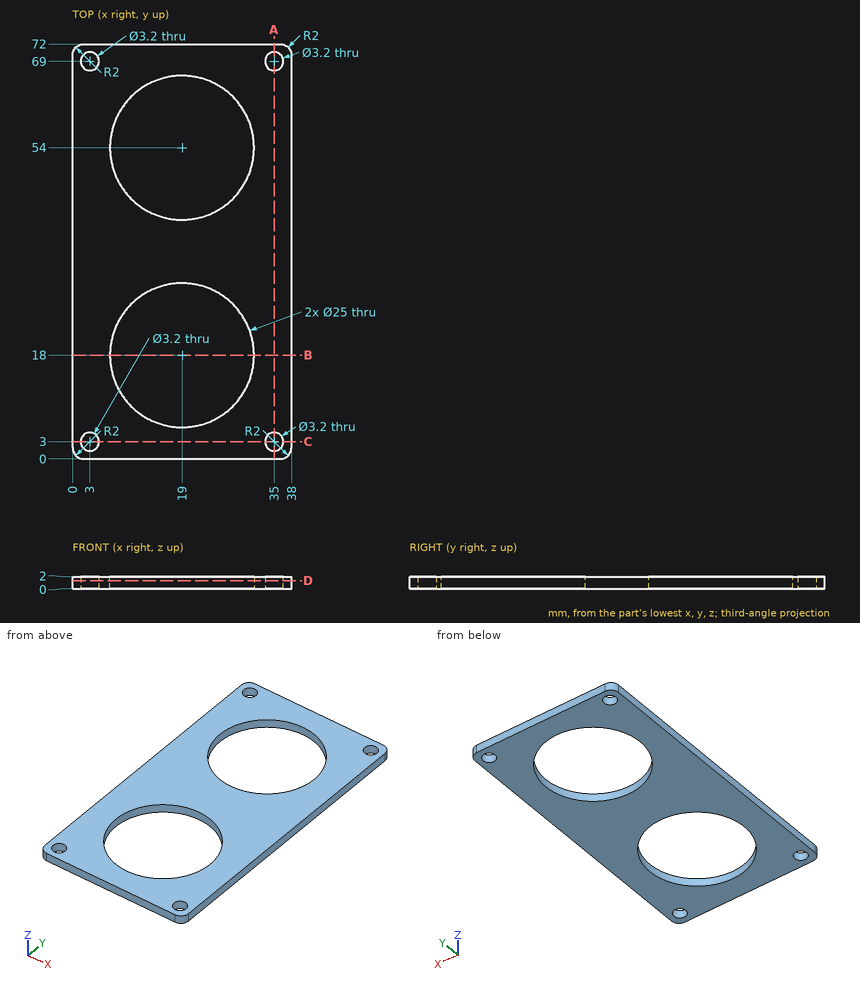
Input: dimensioned drawing with shaded views. Units: mm. Origin: part minimum x, y, z. Give positions to 0.01 mm unless a question says otherwise; leave off trailing zeros. Loops run counter-clockwise (first coordinate to the right, second up) from the corner with the lowest first, then second, coordinate; pieces in that order, holes last. Notation, with made-up numbers: (37.25, -40) -> (60.25, -40) arc R10 cw to (60.25, -30) -> close; hole circle Ø3 at (-11, 58.25). An arc over 180 degrees is marked (long way). Use a Markdown table: item, result. Add a question column.
1) Line query: line 1 along Y through (x, z) = (3, 1.3); line 2 along Y through (x, z) = (19, 1.3); line 3 along X through (y, z) = (69, 0.95). Output: solid intervals per line, ascending. Write a range as [from, to].
2) Section query B-B, the plane y = 18. Return the cut outline in (x, z).
3) First-contact query: pin 1 (3.5 mm diameter, centred on x = 3, y = 3, fed in from -Z). Flat tip, straight axial feed; report the tip coordinate or a pass-through.
4) Section query A-A, the plane x = 35. Return the cut outline in (y, z), then the cut area to 3 significant figures.
5) Section query C-C, the plane y = 3. Return the cut outline in (x, z), then the cut area to 3 significant figures.
6) Section query D-D, the plane z = 1.35. Return the cut outline in (x, y).
Numbers:
| question | item | result |
|---|---|---|
| 1 | line 1 | y = [0, 1.4], [4.6, 67.4], [70.6, 72] |
| 1 | line 2 | y = [0, 5.5], [30.5, 41.5], [66.5, 72] |
| 1 | line 3 | x = [0, 1.4], [4.6, 33.4], [36.6, 38] |
| 2 | outline | (0, 0) -> (6.5, 0) -> (6.5, 2) -> (0, 2) -> close; (31.5, 0) -> (38, 0) -> (38, 2) -> (31.5, 2) -> close |
| 3 | pin 1 | stops at z = 0 |
| 4 | outline | (0, 0) -> (1.4, 0) -> (1.4, 2) -> (0, 2) -> close; (4.6, 0) -> (67.4, 0) -> (67.4, 2) -> (4.6, 2) -> close; (70.6, 0) -> (72, 0) -> (72, 2) -> (70.6, 2) -> close |
| 4 | area | 131 mm2 |
| 5 | outline | (0, 0) -> (1.4, 0) -> (1.4, 2) -> (0, 2) -> close; (4.6, 0) -> (33.4, 0) -> (33.4, 2) -> (4.6, 2) -> close; (36.6, 0) -> (38, 0) -> (38, 2) -> (36.6, 2) -> close |
| 5 | area | 63.2 mm2 |
| 6 | outline | (0, 2) arc R2 ccw to (2, 0) -> (36, 0) arc R2 ccw to (38, 2) -> (38, 70) arc R2 ccw to (36, 72) -> (2, 72) arc R2 ccw to (0, 70) -> close; hole circle Ø3.2 at (3, 3); hole circle Ø3.2 at (3, 69); hole circle Ø25 at (19, 18); hole circle Ø25 at (19, 54); hole circle Ø3.2 at (35, 3); hole circle Ø3.2 at (35, 69) |
